For this review, take the finished solid that the model builds, in its own axes (mm). A direction names the side the tool comes from. Coordinates: 2 decimals unless noted, no trailing zeros. Order: outer loops, then holes, each group sorted by start corner. A loop starts at its lowest first (then second) coordinate and runs counter-clockwise, first axis right, second up. Notation, with made-up numbers: (12.5, 14) - (42.5, 14) arc R25 ccw to (42.5, 44) - close; hole circle Ø10 at (82, 9). An arc over 180 degrees is marked (long way). One line per item, written item: value. Start each with the question number.
(1) Mouldability with a two-part tool opening along Z and no side actions: class faces 4 (the flat face through (66.675, 5, 7)), 5 (the cylindrical face through (67.595, 4.829, -7.423)), 6 (the flat face through (-60, 5, 9.462)) as released by +Z, released by -Z, zero draft, split by the parting line, or undercut.
(2) Consider section A-A on z = 6.35. Write out the cut boundary in (x, y) (3 decimals).
(3) To check wall thickness, follow line 1 along X through (y, z) = (3.5, 6.35) (3 decimals); line 2 along X through (y, z) = (0.5, 3) (3 decimals); line 3 along X through (y, z) = (5, 4) (3 decimals). State the ranges of each line that lie inside material, in increasing order.
(4) Clearance check with flat-ended pins moving along their axes: pin 1 (17.5 mm diameter, centred on x = 39.9, z = 6.35, fed in from +Y); pin 2 (1.9 mm diameter, centred on x = 73, y = 5.5, fed in from +Z); pin 3 (2 mm diameter, centred on y = 3.5, z = -14.5, fed in from +X); pin 4 (4 mm diameter, centred on x = -61, y = 5, fed in from -Z). State where each tip first meets the part, or that it passes through.
(5) For faces 1 (the flat face through (73, 5, -6.477)), 2 (the flat face through (-53.975, 5, 15)), 3 (the cylindrical face through (-26.177, 4.829, -2.21)), list the 3-axis set-ups (+Z, -Z, +X, -X, +Y, -Y) from which the entire face can be reached by the end or side of a thin tool; tool diameter is ignored.
(6) Consider section B-B on x = -14.5. Write out the cut boundary in (y, z) (3 decimals), then the cut area to 3 significant figures.
```python
from build123d import *

# Parameters (mm, degrees)
SKETCH1_W           = 127
SKETCH1_H           = 38.1
BOSS_EXTRUDE1_DEPTH = 9.525
CUT_EXTRUDE2_DEPTH  = 10.525
SKETCH4_R           = 2.2225
CUT_EXTRUDE3_DEPTH  = 10.525
SKETCH5_R           = 3.1115
CUT_EXTRUDE4_DEPTH  = 2.5
SKETCH7_R           = 1.3890625
CUT_EXTRUDE6_DEPTH  = 10.525
SKETCH8_R           = 11.0363
CUT_EXTRUDE7_DEPTH  = 10.525
SKETCH9_R           = 1.524
CUT_EXTRUDE8_DEPTH  = 10.525
BOSS_EXTRUDE3_DEPTH = 9.525
SKETCH11_R          = 1.3890625
CUT_EXTRUDE9_DEPTH  = 10.525
CUT_EXTRUDE10_DEPTH = 10.525
SKETCH14_R          = 2.0955
CUT_EXTRUDE11_DEPTH = 10.525
SKETCH15_W          = 9.525
SKETCH15_H          = 25.527
CUT_EXTRUDE12_DEPTH = 10.525
SKETCH16_R          = 2.0955
CUT_EXTRUDE13_DEPTH = 10.525
SKETCH17_R          = 1.524
CUT_EXTRUDE14_DEPTH = 10.525
FILLET1_R           = 0.635


with BuildPart() as part:
    # Sketch1 → Boss-Extrude1 (new body)
    with BuildSketch(Plane(origin=(0, 0, 0), x_dir=(1, 0, 0), z_dir=(0, 1, 0))):
        Rectangle(SKETCH1_W, SKETCH1_H)
    extrude(amount=BOSS_EXTRUDE1_DEPTH)

    # Sketch3 → Cut-Extrude2 (cut, through all)
    with BuildSketch(Plane.XZ):
        Polygon((0, -19.05), (-63.5, -12.7), (-63.5, -19.05), align=None)
    extrude(amount=-CUT_EXTRUDE2_DEPTH, mode=Mode.SUBTRACT)

    # Sketch4 → Cut-Extrude3 (cut, through all)
    with BuildSketch(Plane(origin=(0, 9.525, 0), x_dir=(1, 0, 0), z_dir=(0, 1, 0))):
        with Locations((-39.9034, -6.35)):
            Circle(SKETCH4_R)
        with Locations((39.9034, -6.35)):
            Circle(SKETCH4_R)
    extrude(amount=-CUT_EXTRUDE3_DEPTH, mode=Mode.SUBTRACT)

    # Sketch5 → Cut-Extrude4 (cut)
    with BuildSketch(Plane(origin=(0, 9.525, 0), x_dir=(1, 0, 0), z_dir=(0, 1, 0))):
        with Locations((-39.9034, -6.35)):
            Circle(SKETCH5_R)
        with Locations((39.9034, -6.35)):
            Circle(SKETCH5_R)
    extrude(amount=-CUT_EXTRUDE4_DEPTH, mode=Mode.SUBTRACT)

    # Sketch7 → Cut-Extrude6 (cut, through all)
    with BuildSketch(Plane.XZ):
        with Locations((-58.7375, -7.9375)):
            Circle(SKETCH7_R)
        with Locations((-58.7375, 14.2875)):
            Circle(SKETCH7_R)
    extrude(amount=-CUT_EXTRUDE6_DEPTH, mode=Mode.SUBTRACT)

    # Sketch8 → Cut-Extrude7 (cut, through all)
    with BuildSketch(Plane(origin=(0, 9.525, 0), x_dir=(1, 0, 0), z_dir=(0, 1, 0))):
        with Locations((-39.9034, -6.35)):
            Circle(SKETCH8_R)
        with Locations((39.9034, -6.35)):
            Circle(SKETCH8_R)
    extrude(amount=-CUT_EXTRUDE7_DEPTH, mode=Mode.SUBTRACT)

    # Sketch9 → Cut-Extrude8 (cut, through all)
    with BuildSketch(Plane(origin=(0, 9.525, 0), x_dir=(1, 0, 0), z_dir=(0, 1, 0))):
        with Locations((0, 8.255)):
            Circle(SKETCH9_R)
    extrude(amount=-CUT_EXTRUDE8_DEPTH, mode=Mode.SUBTRACT)

    # Sketch10 → Boss-Extrude3 (add, through all)
    with BuildSketch(Plane(origin=(0, 9.525, 0), x_dir=(1, 0, 0), z_dir=(0, 1, 0))):
        Polygon((63.5, -19.05), (63.5, 19.05), (76.2, 6.35), (76.2, -19.05), align=None)
    extrude(amount=-BOSS_EXTRUDE3_DEPTH)

    # Sketch11 → Cut-Extrude9 (cut, through all)
    with BuildSketch(Plane(origin=(0, 9.525, 0), x_dir=(1, 0, 0), z_dir=(0, 1, 0))):
        with Locations((71.4375, 1.5875)):
            Circle(SKETCH11_R)
        with Locations((71.4375, -14.2875)):
            Circle(SKETCH11_R)
    extrude(amount=-CUT_EXTRUDE9_DEPTH, mode=Mode.SUBTRACT)

    # Sketch13 → Cut-Extrude10 (cut, through all)
    with BuildSketch(Plane(origin=(0, 9.525, 0), x_dir=(1, 0, 0), z_dir=(0, 1, 0))):
        Polygon((-63.5, -19.05), (-53.975, -19.05), (-53.975, -9.4615), (-63.5, -9.4615), (-63.5, -14.2875), align=None)
        Polygon((-63.5, 12.7), (-63.5, 3.1115), (-53.975, 3.1115), (-53.975, 12.7), (-53.975, 13.6525), align=None)
    extrude(amount=-CUT_EXTRUDE10_DEPTH, mode=Mode.SUBTRACT)

    # Sketch14 → Cut-Extrude11 (cut, through all)
    with BuildSketch(Plane(origin=(0, 9.525, 0), x_dir=(1, 0, 0), z_dir=(0, 1, 0))):
        with Locations((-55.860468878, 4.0259)):
            Circle(SKETCH14_R)
        with Locations((-55.860468878, -10.3759)):
            Circle(SKETCH14_R)
    extrude(amount=-CUT_EXTRUDE11_DEPTH, mode=Mode.SUBTRACT)

    # Sketch15 → Cut-Extrude12 (cut, through all)
    with BuildSketch(Plane(origin=(0, 9.525, 0), x_dir=(1, 0, 0), z_dir=(0, 1, 0))):
        with Locations((71.4375, -6.2865)):
            Rectangle(SKETCH15_W, SKETCH15_H)
    extrude(amount=-CUT_EXTRUDE12_DEPTH, mode=Mode.SUBTRACT)

    # Sketch16 → Cut-Extrude13 (cut, through all)
    with BuildSketch(Plane(origin=(0, 9.525, 0), x_dir=(1, 0, 0), z_dir=(0, 1, 0))):
        with Locations((68.560468878, 5.5626)):
            Circle(SKETCH16_R)
    extrude(amount=-CUT_EXTRUDE13_DEPTH, mode=Mode.SUBTRACT)

    # Sketch17 → Cut-Extrude14 (cut, through all)
    with BuildSketch(Plane(origin=(0, 9.525, 0), x_dir=(1, 0, 0), z_dir=(0, 1, 0))):
        with Locations((-54.912865865, -3.175)):
            Circle(SKETCH17_R)
        with Locations((-27.5844, 2.793682494)):
            Circle(SKETCH17_R)
        with Locations((-27.5844, -15.493682494)):
            Circle(SKETCH17_R)
        with Locations((27.5844, -15.493682494)):
            Circle(SKETCH17_R)
        with Locations((27.5844, 2.793682494)):
            Circle(SKETCH17_R)
        with Locations((52.2224, 2.793682494)):
            Circle(SKETCH17_R)
        with Locations((52.2224, -15.493682494)):
            Circle(SKETCH17_R)
    extrude(amount=-CUT_EXTRUDE14_DEPTH, mode=Mode.SUBTRACT)

    # Fillet1
    fillet1_edges = [part.edges().sort_by_distance(p)[0] for p in [
        (-63.5, 4.7625, 9.4615),
        (-53.975, 4.7625, 19.05),
        (-53.975, 4.7625, -13.6525),
        (-63.5, 4.7625, -3.1115),
        (-53.975, 4.7625, 11.2903),
        (-57.745937756, 4.7625, -3.1115),
        (-53.975, 4.7625, -4.9403),
        (-57.745937756, 4.7625, 9.4615),
        (76.073, 4.7625, -6.477),
        (66.675, 4.7625, 19.05),
        (0, 4.7625, -19.05),
        (70.445937756, 4.7625, -6.477),
        (66.675, 4.7625, -4.6482),
        (63.5, 4.7625, -19.05),
    ]]
    fillet(fillet1_edges, radius=FILLET1_R)


solid = part.part
```
Geometry check:
1. face 4: zero draft
1. face 5: undercut
1. face 6: released by +Z
2. outline: (-63.5, 0) - (-50.94, 0) - (-50.94, 9.525) - (-63.5, 9.525) - close; (-28.867, 0) - (28.867, 0) - (28.867, 9.525) - (-28.867, 9.525) - close; (50.94, 0) - (66.675, 0) - (66.675, 9.525) - (50.94, 9.525) - close
3. line 1: x = -63.5 to -50.94, -28.867 to 28.867, 50.94 to 66.675
3. line 2: x = -63.5 to -56.427, -53.399 to -50.419, -29.388 to 29.388, 50.419 to 66.675
3. line 3: x = -63.5 to -56.194, -53.631 to -50.687, -29.12 to 29.12, 50.687 to 66.675
4. pin 1: passes through
4. pin 2: stops at z = -6.48
4. pin 3: stops at x = 69.05
4. pin 4: stops at z = -3.11
5. face 1: +Z, +X, +Y, -Y
5. face 2: +Z, -X, +Y, -Y
5. face 3: +Y, -Y
6. outline: (0, -17.6) - (9.525, -17.6) - (9.525, 19.05) - (0, 19.05) - close
6. area: 349 mm^2
